from build123d import *

# Parameters (mm, degrees)
SKETCH1_W                        = 222.5
SKETCH1_H                        = 80
BOSS_EXTRUDE1_DEPTH              = 6.35
SKETCH6_W                        = 6.35
SKETCH6_H                        = 40
CUT_EXTRUDE3_DEPTH               = 12.7
M3_5X0_6_TAPPED_HOLE1_AT_2_COUNT = 2
M3_5X0_6_TAPPED_HOLE1_AT_2_PITCH = 15
CUT_EXTRUDE1_DEPTH               = 119.392926309
CUT_EXTRUDE2_DEPTH               = 119.392926309
M5_CLEARANCE_HOLE1_D             = 5.3
FILLET1_R                        = 7


with BuildPart() as part:
    # Sketch1 → Boss-Extrude1 (new body)
    with BuildSketch(Plane.XY):
        Rectangle(SKETCH1_W, SKETCH1_H)
    extrude(amount=BOSS_EXTRUDE1_DEPTH)

    # Sketch6 → Cut-Extrude3 (cut)
    with BuildSketch(Plane.ZY.offset(111.25)):
        with Locations((3.175, -20)):
            Rectangle(SKETCH6_W, SKETCH6_H)
    cut_extrude3 = extrude(amount=-CUT_EXTRUDE3_DEPTH, mode=Mode.SUBTRACT)

    # Sketch7 → M3.5x0.6 Tapped Hole1 (revolve, cut)
    with BuildSketch(Plane(origin=(-98.55, -25, 3.175), x_dir=(0, 0, 1), z_dir=(0, 1, 0))):
        Polygon((0, 0), (0, 14.671247898), (1.45, 13.8), (1.45, 0), align=None)
    m3_5x0_6_tapped_hole1 = revolve(axis=Axis((-104.9, -25, 3.175), (1, 0, 0)), mode=Mode.SUBTRACT)

    # M3.5x0.6 Tapped Hole1 at 2: M3.5x0.6 Tapped Hole1 ×2
    with Locations(*[(0, i * M3_5X0_6_TAPPED_HOLE1_AT_2_PITCH, 0) for i in range(1, M3_5X0_6_TAPPED_HOLE1_AT_2_COUNT)]):
        add(m3_5x0_6_tapped_hole1, mode=Mode.SUBTRACT)

    # Sketch2 → Cut-Extrude1 (cut, through all)
    with BuildSketch(Plane.XY.offset(6.35)):
        Polygon((111.25, 40), (0, -0.491688562), (-111.25, 40), align=None)
    extrude(amount=-CUT_EXTRUDE1_DEPTH, mode=Mode.SUBTRACT)

    # Sketch3 → Cut-Extrude2 (cut, through all)
    with BuildSketch(Plane.XY.offset(6.35)):
        Polygon((-87.25, -33), (-87.25, 18.494581108), (-6, -11.078000426), (-6, -33), align=None)
    cut_extrude2 = extrude(amount=-CUT_EXTRUDE2_DEPTH, mode=Mode.SUBTRACT)

    # M5 Clearance Hole1 (through all)
    with Locations(Plane(origin=(0, 0, 0), x_dir=(-1, 0, 0), z_dir=(0, 0, -1))):
        with Locations((104.9, 10), (104.9, 25)):
            m5_clearance_hole1 = Hole(M5_CLEARANCE_HOLE1_D / 2)

    # Mirror1: Cut-Extrude3, M3.5x0.6 Tapped Hole1, Cut-Extrude2, M5 Clearance Hole1 across plane
    add(cut_extrude3.mirror(Plane(origin=(0, 0, 0), x_dir=(0, 0, 1), z_dir=(1, 0, 0))), mode=Mode.SUBTRACT)
    add(m3_5x0_6_tapped_hole1.mirror(Plane(origin=(0, 0, 0), x_dir=(0, 0, 1), z_dir=(1, 0, 0))), mode=Mode.SUBTRACT)
    add(cut_extrude2.mirror(Plane(origin=(0, 0, 0), x_dir=(0, 0, 1), z_dir=(1, 0, 0))), mode=Mode.SUBTRACT)
    add(m5_clearance_hole1.mirror(Plane(origin=(0, 0, 0), x_dir=(0, 0, 1), z_dir=(1, 0, 0))), mode=Mode.SUBTRACT)

    # Mirror1 copy 1 sketch → Mirror1 copy 1 (revolve, cut)
    with BuildSketch(Plane(origin=(98.55, -10, 3.175), x_dir=(0, 0, 1), z_dir=(0, 1, 0))):
        Polygon((0, 0), (0, -14.671247898), (1.45, -13.8), (1.45, 0), align=None)
    revolve(axis=Axis((104.9, -10, 3.175), (1, 0, 0)), mode=Mode.SUBTRACT)

    # Fillet1
    fillet1_edges = [part.edges().sort_by_distance(p)[0] for p in [
        (87.25, 18.494581108, 3.175),
        (87.25, -33, 3.175),
        (6, -33, 3.175),
        (6, -11.078000426, 3.175),
        (-98.55, -40, 3.175),
        (-111.25, 0, 3.175),
        (0, -0.491688562, 3.175),
        (-87.25, -33, 3.175),
        (-6, -33, 3.175),
        (-87.25, 18.494581108, 3.175),
        (-6, -11.078000426, 3.175),
        (-111.25, 40, 3.175),
        (111.25, 40, 3.175),
        (111.25, 0, 3.175),
        (98.55, -40, 3.175),
    ]]
    fillet(fillet1_edges, radius=FILLET1_R)


solid = part.part
The model under review builds one solid part; all positions refer to its coordinate system, in mm. A direction names the side the tool comes from. Give positions to 0.01 mm unless a question says otherwise; leave off trailing zeros. Loops run counter-clockwise (first coordinate to the right, second up) from the corner with the lowest first, then second, coordinate; pieces in that order, holes last. Notation, with made-up numbers: (78.5, 60.5) -> (83.5, 60.5) arc R21 ccw to (83.5, 97.5) -> close; hole circle Ø11 at (66.5, 23). An arc over 180 degrees is marked (long way). Put each result on its own line as item: value. Start each with the question number.
1. We need section D-D on y = -31. State how many separate pieces and enclosed holes the cut face has, then the cut area to 3 significant figures.
2. Wall thickness on probe 1 along Y at (x, z) = (-104.9, 2); probe 2 along X at (y, z) = (-27.5, 2); probe 3 along X at (y, z) = (-26, 0.5): over which ranges is each line inside the solid? List them lowest first.
3. We need section A-A on y = 3.5. State the section outline as (x, z) points.
4. For faces 1 (the face through (101, 0, 3)), 2 (the face through (-85.15, -31, 5.27)), 3 (the face through (-108.342, 35.683, 3.219)), list the 3-axis set-ups (+Z, -Z, +X, -X, +Y, -Y) from which the entire face can be reached by the end or side of a thin tool; tool diameter is ignored.
5. We need section B-B on x = 59. State the section outline as (y, z) points, then the cut area to 3 significant figures.
6. Clearance check with flat-ended pins moving along their axes: P1, Ø10, axis at x = -80, y = -18, coming from the -Z side; P2, Ø1.5, axis at y = -29.5, z = 3.5, coming from the -X side; P3, Ø1.9, axis at x = -55.5, z = 4.5, coming from the +Y side; P4, Ø1.7, axis at y = -25, z = 3.175, coming from the -X side. State where each tip first meets the part, or that it passes through.
7. Mouldability with a two-part tool opening along Y and no side actions: class faces 4 (the face through (23, -1, 0)), 5 (the face through (96.45, -38, 3.22)), 6 (the face through (-85.15, -31, 1.05)) as released by +Y, released by -Y, zero draft, split by the parting line, or undercut.
8. We need section C-C on x = -8.5. State the section outline as (y, z) points, then the cut area to 3 significant figures.
Determined:
1. separate pieces: 3
1. enclosed holes: 0
1. area: 273 mm^2
2. probe 1: 0.03 to 7.35, 12.65 to 22.35, 27.65 to 36.97
2. probe 2: -98.55 to -87.09, -6.16 to 6.16, 87.09 to 98.55
2. probe 3: -98.55 to -87.25, -6 to 6, 87.25 to 98.55
3. outline: (-110.31, 0) -> (-87.25, 0) -> (-87.25, 6.35) -> (-110.31, 6.35) -> close; (-46.05, 0) -> (-10.97, 0) -> (-10.97, 6.35) -> (-46.05, 6.35) -> close; (10.97, 0) -> (46.05, 0) -> (46.05, 6.35) -> (10.97, 6.35) -> close; (87.25, 0) -> (110.31, 0) -> (110.31, 6.35) -> (87.25, 6.35) -> close
4. face 1: +Z, -Z, +X, -Y
4. face 2: +Z, -Z
4. face 3: +Z, -Z, +Y
5. outline: (-40, 0) -> (-33, 0) -> (-33, 6.35) -> (-40, 6.35) -> close; (8.21, 0) -> (20.98, 0) -> (20.98, 6.35) -> (8.21, 6.35) -> close
5. area: 126 mm^2
6. P1: through
6. P2: x = -98.55
6. P3: y = 20.05
6. P4: x = -6
7. face 4: zero draft
7. face 5: released by -Y
7. face 6: undercut
8. outline: (-40, 0) -> (-31.36, 0) -> (-31.36, 6.35) -> (-40, 6.35) -> close; (-10.62, 0) -> (2.6, 0) -> (2.6, 6.35) -> (-10.62, 6.35) -> close
8. area: 139 mm^2
